from build123d import *

# Parameters (mm, degrees)
SKETCH1_W             = 51.5
SKETCH1_H             = 37.5
BOSS_EXTRUDE1_DEPTH   = 40
SKETCH2_W             = 49.5
SKETCH2_H             = 38
CUT_EXTRUDE1_DEPTH    = 61.574850392
FILLET1_R             = 1
FILLET2_R             = 2
F_3_0MM_DOWEL_HOLE1_D = 3
CUT_EXTRUDE2_DEPTH    = 10
FILLET3_R             = 18.75
F_3_0MM_DOWEL_HOLE2_D = 3


with BuildPart() as part:
    # Sketch1 → Boss-Extrude1 (new body)
    with BuildSketch(Plane(origin=(0, 0, 0), x_dir=(1, 0, 0), z_dir=(0, 1, 0))):
        Rectangle(SKETCH1_W, SKETCH1_H)
    extrude(amount=BOSS_EXTRUDE1_DEPTH)

    # Sketch2 → Cut-Extrude1 (cut, through all)
    with BuildSketch(Plane.XY.offset(18.75)):
        with Locations((1, 21)):
            Rectangle(SKETCH2_W, SKETCH2_H)
    extrude(amount=-CUT_EXTRUDE1_DEPTH, mode=Mode.SUBTRACT)

    # Fillet1
    fillet1_edges = [part.edges().sort_by_distance(p)[0] for p in [
        (-23.75, 2, 0),
    ]]
    fillet(fillet1_edges, radius=FILLET1_R)

    # Fillet2
    fillet2_edges = [part.edges().sort_by_distance(p)[0] for p in [
        (-25.75, 0, 0),
    ]]
    fillet(fillet2_edges, radius=FILLET2_R)

    # Ø3.0mm Dowel Hole1 (through all)
    with Locations(Plane(origin=(0, 2, 0), x_dir=(1, 0, 0), z_dir=(0, 1, 0))):
        with Locations((-17.15, -15.575), (-17.15, 15.575), (-10.85, -15.575), (-4.55, -15.575), (1.75, -15.575), (8.05, -15.575), (14.35, -15.575), (20.65, -15.575), (20.65, 15.575), (14.35, 15.575), (8.05, 15.575), (1.75, 15.575), (-4.55, 15.575), (-10.85, 15.575)):
            Hole(F_3_0MM_DOWEL_HOLE1_D / 2)

    # Sketch7 → Cut-Extrude2 (cut)
    with BuildSketch(Plane.ZY.offset(25.75)):
        with BuildLine():
            Line((6.6, 27.246787517), (6.6, 13.6))
            ThreePointArc((6.6, 13.6), (0, 7), (-6.6, 13.6))
            Line((-6.6, 13.6), (-6.6, 27.246787517))
            ThreePointArc((-6.6, 27.246787517), (0, 33.846787517), (6.6, 27.246787517))
        make_face()
    extrude(amount=-CUT_EXTRUDE2_DEPTH, mode=Mode.SUBTRACT)

    # Fillet3
    fillet3_edges = [part.edges().sort_by_distance(p)[0] for p in [
        (-24.75, 40, 18.75),
        (-24.75, 40, -18.75),
    ]]
    fillet(fillet3_edges, radius=FILLET3_R - 0.0001)  # a hair under: the kernel refuses the full size

    # Ø3.0mm Dowel Hole2 (through all)
    with Locations(Plane.ZY.offset(25.75)):
        with Locations((-7.75, 33.846787517), (7.75, 33.846787517), (15.5, 20.423393759), (7.75, 7), (-7.75, 7), (-15.5, 20.423393759)):
            Hole(F_3_0MM_DOWEL_HOLE2_D / 2)


solid = part.part
Can you work these out from the model? Positions are in its coordinate system, mm. A direction names the side the tool comes from. Coordinates: 2 decimals unless noted, no trailing zeros. Write each loop counter-clockwise with the first axis right and the second up, starting at its lowest first coordinate (ties: lowest second). Pieces come first, ordered by that corner, then holes. Notation, with made-up numbers: (-8.5, 38.25) -> (8.5, 38.25) arc R23 cw to (8.5, 67.25) -> close; hole circle Ø1 at (59.25, 64). An arc over 180 degrees is marked (long way). Write each question's results on one line, items separated by ' | '. Start each with the question number.
Item 1: If we section it at C-C, the plane z = 3: Write out the boundary of the cut face in (x, y), and give its area (3 significant figures).
Item 2: Please list where these lines run through material, in increasing order: probe 1 along Y at (x, z) = (-20, -13); probe 2 along Y at (x, z) = (-24.5, 7.75); probe 3 along X at (y, z) = (12, 15).
Item 3: On a 3-axis mill with a long thin cutter (end or side, diameter ignored), from which of +Z, -Z, +X, -X, +Y, -Y can I reach the whole of each face in a straight line? I mean faces 1 (the flat face through (-25, 20, -6.6)), 2 (the cylindrical face through (-17.842, 0.986, 16.906)), 3 (the flat face through (-23.75, 21, -8)). Say none if no direction works.
Item 4: I'm going to push flat-ended pins straight in: P1, Ø5, axis at x = -17.15, z = 15.575, coming from the +Y side; P2, Ø5, axis at y = 7, z = 7.75, coming from the +X side; P3, Ø1, axis at x = 7.5, z = -0.5, coming from the -Y side. Where does each tip first touch, or does it pass through?
Item 5: If we section it at A-A, the plane x = 8.05: Write out the boundary of the cut face in (y, z) (3 decimals), and give its area (3 significant figures).
Item 6: If we section it at B-B, the plane y = 14.5: Write out the boundary of the cut face in (x, z).
Item 7: If we section it at D-D, the plane z = 7.75: Write out the boundary of the cut face in (x, y), and give its area (3 significant figures).
Item 8: Thinking about a two-plate mould opening in Z: for faces 4 (the cylindrical face through (21.84, 0.99, 16.49)), 5 (the flat face through (1, 2, 0)), 6 (the flat face through (-6, 1, 18.75)), 7 (the flat face through (-6, 1, -18.75)), which applies, released by +Z, released by -Z, zero draft, split by the parting line, or undercut?
Answer block:
1) outline: (-25.75, 2) arc R2 ccw to (-23.75, 0) -> (25.75, 0) -> (25.75, 2) -> (-22.75, 2) arc R1 cw to (-23.75, 3) -> (-23.75, 7.72) -> (-25.75, 7.72) -> close; (-25.75, 33.13) -> (-23.75, 33.13) -> (-23.75, 39.76) -> (-25.75, 39.76) -> close | area: 127 mm²
2) probe 1: 0 to 2 | probe 2: 0.15 to 5.5, 8.5 to 32.35, 35.35 to 38.32 | probe 3: -25.75 to -23.75
3) face 1: +X, -X | face 2: +Y, -Y | face 3: +Z, -Z, +X, +Y
4) P1: y = 2 | P2: x = -23.75 | P3: y = 0
5) outline: (0, -18.75) -> (2, -18.75) -> (2, -17.075) -> (0, -17.075) -> close; (0, -14.075) -> (2, -14.075) -> (2, 14.075) -> (0, 14.075) -> close; (0, 17.075) -> (2, 17.075) -> (2, 18.75) -> (0, 18.75) -> close | area: 63.0 mm²
6) outline: (-25.75, -18.75) -> (-23.75, -18.75) -> (-23.75, -6.6) -> (-25.75, -6.6) -> close; (-25.75, 6.6) -> (-23.75, 6.6) -> (-23.75, 18.75) -> (-25.75, 18.75) -> close
7) outline: (-25.75, 2) arc R2 ccw to (-23.75, 0) -> (25.75, 0) -> (25.75, 2) -> (-22.75, 2) arc R1 cw to (-23.75, 3) -> (-23.75, 5.5) -> (-25.75, 5.5) -> close; (-25.75, 8.5) -> (-23.75, 8.5) -> (-23.75, 32.35) -> (-25.75, 32.35) -> close; (-25.75, 35.35) -> (-23.75, 35.35) -> (-23.75, 38.32) -> (-25.75, 38.32) -> close | area: 163 mm²
8) face 4: undercut | face 5: zero draft | face 6: released by +Z | face 7: released by -Z
